```python
from build123d import *

# Parameters (mm, degrees)
SKETCH2_W                                           = 240
SKETCH2_H                                           = 180
EXTRUDE1_DEPTH                                      = 20
CBORE_FOR_M5_HEX_SOCKET_HEAD_CAP_SCREW1_D           = 5.5
CBORE_FOR_M5_HEX_SOCKET_HEAD_CAP_SCREW1_DEPTH       = 29
CBORE_FOR_M5_HEX_SOCKET_HEAD_CAP_SCREW1_CBORE_D     = 10
CBORE_FOR_M5_HEX_SOCKET_HEAD_CAP_SCREW1_CBORE_DEPTH = 5.4
CBORE_FOR_M5_HEX_SOCKET_HEAD_CAP_SCREW1_TIP         = 1.652366702
M6_TAPPED_HOLE1_D                                   = 5
CBORE_FOR_M6_HEX_SOCKET_HEAD_CAP_SCR_2_COUNT        = 2
CBORE_FOR_M6_HEX_SOCKET_HEAD_CAP_SCR_2_PITCH        = 35


with BuildPart() as part:
    # Sketch2 → Extrude1 (new body)
    with BuildSketch(Plane.XY):
        Rectangle(SKETCH2_W, SKETCH2_H)
    extrude(amount=EXTRUDE1_DEPTH)

    # CBORE for M5 Hex Socket Head Cap Screw1
    with Locations(Plane.XY.offset(20)):
        with Locations((-101.5, 75.6), (-63.5, 75.6), (-63.5, 45.6), (-101.5, 45.6), (63.5, 75.6), (101.5, 75.6), (101.5, 45.6), (63.5, 45.6), (101.5, -45.6), (63.5, -45.6), (63.5, -75.6), (101.5, -75.6), (-63.5, -75.6), (-63.5, -45.6), (-101.5, -45.6), (-101.5, -75.6)):
            CounterBoreHole(CBORE_FOR_M5_HEX_SOCKET_HEAD_CAP_SCREW1_D / 2, CBORE_FOR_M5_HEX_SOCKET_HEAD_CAP_SCREW1_CBORE_D / 2, CBORE_FOR_M5_HEX_SOCKET_HEAD_CAP_SCREW1_CBORE_DEPTH, depth=CBORE_FOR_M5_HEX_SOCKET_HEAD_CAP_SCREW1_DEPTH)
            with Locations((0, 0, -(CBORE_FOR_M5_HEX_SOCKET_HEAD_CAP_SCREW1_DEPTH + CBORE_FOR_M5_HEX_SOCKET_HEAD_CAP_SCREW1_TIP / 2))):  # 118° drill point
                Cone(0, CBORE_FOR_M5_HEX_SOCKET_HEAD_CAP_SCREW1_D / 2, CBORE_FOR_M5_HEX_SOCKET_HEAD_CAP_SCREW1_TIP, mode=Mode.SUBTRACT)

    # M6 Tapped Hole1 (through all)
    with Locations(Plane.XY.offset(20)):
        with Locations((-90, 75), (90, 75), (90, -15), (90, -75), (-90, -15), (-90, -75)):
            Hole(M6_TAPPED_HOLE1_D / 2)

    # Sketch8 → CBORE for M6 Hex Socket Head Cap Screw1 (revolve, cut)
    with BuildSketch(Plane(origin=(17.5, -21.2, 20), x_dir=(0, -1, 0), z_dir=(1, 0, 0))):
        Polygon((0, 0), (0, 13.482840043), (3.3, 11.5), (3.3, 6.4), (5.5, 6.4), (5.5, 0.025), (5.525, 0), align=None)
    cbore_for_m6_hex_socket_head_cap_screw1 = revolve(axis=Axis((17.5, -21.2, 26.35), (0, 0, -1)), mode=Mode.SUBTRACT)

    # CBORE for M6 Hex Socket Head Cap Scr 2: CBORE for M6 Hex Socket Head Cap Screw1 ×2
    with Locations(*[(-i * CBORE_FOR_M6_HEX_SOCKET_HEAD_CAP_SCR_2_PITCH, 0, 0) for i in range(1, CBORE_FOR_M6_HEX_SOCKET_HEAD_CAP_SCR_2_COUNT)]):
        add(cbore_for_m6_hex_socket_head_cap_screw1, mode=Mode.SUBTRACT)


solid = part.part
```
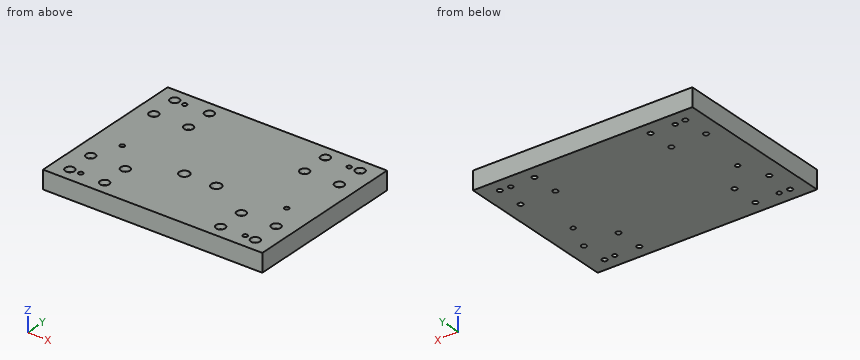
Check sheet for the modelled part. Datum: model origin and axes. Units: mm. Round coordinates to 2 decimals unless told otherwise and drop trailing zeros. Order: outer loops, then holes, each group sorted by start corner. A loop starts at its lowest first (then second) coordinate and runs counter-clockwise, first axis right, second up. Notation, with made-up numbers: (-16, 71.5) - (16, 71.5) arc R22 ccw to (16, 101.5) - close; hole circle Ø2 at (-29.5, 86.5). An arc over 180 degrees is marked (long way). Answer as CSV lines item,"result". Start each with the question number.
1) Section check A-A (x = 90). Record the cut outline in (y, z).
2) Section check B-B (x = -101.5). Give the number of separate pieces and of enclosed holes in the cut face, then the cut area to 3 significant figures.
3) Depth check by flat-ended pin: pin 1 (4.5 mm diameter, centred on x = -63.5, y = -75.6, fed in from -Z); pin 2 (5 mm diameter, centred on x = -103.5, y = -76, fed in from +Z); pin 3 (10.5 mm diameter, centred on x = 17.5, y = -21.2, fed in from +Z). Enter the tip coordinate at first touch or a pass-through.
4) Scan lines: probe 1 along Y at (x, z) = (90, 6); probe 2 along Y at (x, z) = (-63.5, 16.4); probe 3 along X at (y, z) = (-21.2, 16). Record each from-to range of solid material in increasing order.
Determined:
1,outline,"(-90, 0) - (-77.5, 0) - (-77.5, 20) - (-90, 20) - close; (-72.5, 0) - (-17.5, 0) - (-17.5, 20) - (-72.5, 20) - close; (-12.5, 0) - (72.5, 0) - (72.5, 20) - (-12.5, 20) - close; (77.5, 0) - (90, 0) - (90, 20) - (77.5, 20) - close"
2,separate pieces,"5"
2,enclosed holes,"0"
2,area,"3,060 mm^2"
3,pin 1,"through"
3,pin 2,"z = 14.6"
3,pin 3,"z = 13.6"
4,probe 1,"-90 to -77.5, -72.5 to -17.5, -12.5 to 72.5, 77.5 to 90"
4,probe 2,"-90 to -80.6, -70.6 to -50.6, -40.6 to 40.6, 50.6 to 70.6, 80.6 to 90"
4,probe 3,"-120 to -23, -12 to 12, 23 to 120"
